Check sheet for the drawn part. Datum: minimum x, y, z corner. Units: mm. A direction names the side the tool comes from. Give positions to 0.01 mm unless a question says otherwise; leave off trailing zeros. Write each loop counter-clockwise with the first axis right and the second up, starting at its lowest first coordinate (ties: lowest second). Pieces come first, ordered by that corner, then holes. Notation, with made-up numbers: (33.25, 78) -> (91.25, 78) arc R21 cw to (91.25, 102) -> close; hole circle Ø5 at (-8, 31.25). An arc over 180 degrees is marked (long way). Write item = value, one per line. Start each with the question number.
1. Mould release check, pull along X, two halves, no side actions. Record for the marked faces 1, 2, 3 and 4: pulls with the +X half, pulls with the -X half, needs draft (parallel to the pull), parting line crosses it, or undercut.
2. Cross-section at A-A, the plane x = 18.7. Record the cut outline in (y, z).
3. Set-up check for the marked faces 5 and 6: record each of +Z, -Z, +X, -X, +Y, -Y from which the full face is reachable in a straight line by a thin tool's end or side.
4. Depth check by flat-ended pin: P1, Ø1.5, axis at x = 6, z = 1.5, coming from the -Y side (1 decimal). Enter the tip coordinate at first touch or a pass-through.
5. Cross-section at C-C, the plane y = 18.75. Record the cut outline in (x, z), plus the area to 3 significant figures.
6. Cross-section at B-B, the plane z = 1. Record the cut outline in (x, y).
7. Cross-section at D-D, the plane x = 9. Record the cut outline in (y, z).
8. Thickness scan on line 1 along X through (y, z) = (8, 1.15); line 2 along X through (y, z) = (9.25, 0.25) (1 decimal); line 3 along Y through (x, z) = (17.75, 1.6) (1 decimal). Record the ranges inside material, lowest first.
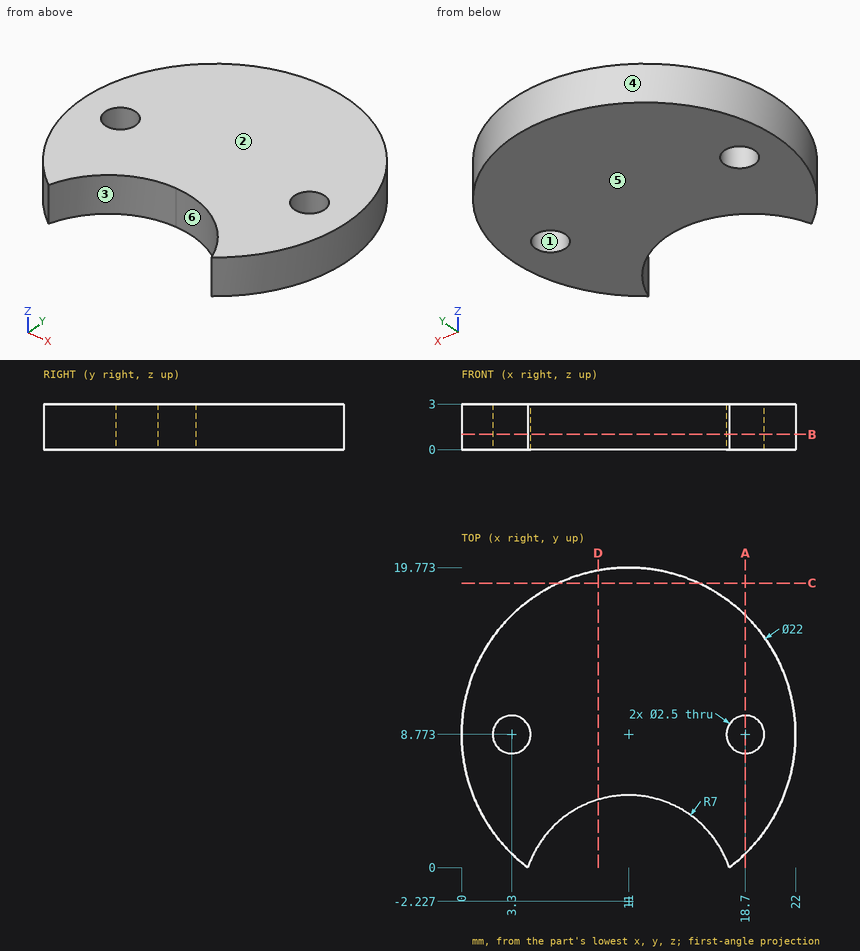
Answers:
q1.face_1 = undercut
q1.face_2 = needs draft
q1.face_3 = undercut
q1.face_4 = parting line crosses it
q2.outline = (0.92, 0) -> (7.52, 0) -> (7.52, 3) -> (0.92, 3) -> close; (10.02, 0) -> (16.63, 0) -> (16.63, 3) -> (10.02, 3) -> close
q3.face_5 = -Z, +X, -X, +Y, -Y
q3.face_6 = +Z, -Z, -Y
q4.P1 = 1.8
q5.outline = (6.37, 0) -> (15.63, 0) -> (15.63, 3) -> (6.37, 3) -> close
q5.area = 27.8 mm^2
q6.outline = (4.36, 0) arc R7 cw to (11, 4.77) arc R7 cw to (17.64, 0) arc R11 ccw (long way) to start; hole circle Ø2.5 at (3.3, 8.77); hole circle Ø2.5 at (18.7, 8.77)
q7.outline = (4.48, 0) -> (19.59, 0) -> (19.59, 3) -> (4.48, 3) -> close
q8.line_1 = 0.03 to 2.32, 4.28 to 17.72, 19.68 to 21.97
q8.line_2 = 0 to 2.1, 4.5 to 17.5, 19.9 to 22
q8.line_3 = 0.1 to 8, 9.6 to 17.5
